Input: part model. Units: mm. Frame: model coordinates. Give positions to 0.01 mm unless a question says otherwise; leave off trailing zeros. Loops run counter-clockwise (first coordinate to the right, second up) from the corner with the lowest first, then second, coordinate; pieces in that order, holes last.
Autodesk Inventor part; units mm, degrees
ref_plane "YZ Plane" through (0, 0, 0) normal (1, 0, 0) x (0, 1, 0)
ref_plane "XZ Plane" through (0, 0, 0) normal (0, 1, 0) x (-1, 0, 0)
ref_plane "XY Plane" through (0, 0, 0) normal (0, 0, 1) x (1, 0, 0)
sketch "main" plane through (0, 0, 0) normal (0, 0, 1) x (1, 0, 0)
  arc A0 (7.9061, 59.9189) -> (2.6576, 57.1432) centre (7.9061, 53.5689) ccw
  line L0 (7.9061, 59.9189) -> (15.7951, 59.9189)
  arc A1 (20.9767, 57.2396) -> (15.7951, 59.9189) centre (15.7951, 53.5689) ccw
  circle A2 centre (15.7951, 53.5689) radius 2.1844
  arc A3 (-27.1814, 13.3264) -> (-31.4423, -3.6797) centre (-6.1872, -0.9705) ccw
  circle A4 centre (15.7951, -9.9311) radius 2.1844
  line L1 (20.9767, 57.2396) -> (20.9767, -12.9584)
  circle A5 centre (-20.2983, -22.6311) radius 2.0955
  line L2 (-2.1836, -39.0438) -> (-15.8326, -52.5455)
  circle A6 centre (-20.2983, -48.0311) radius 2.0955
  line L3 (-31.4423, -3.6797) -> (-26.6121, -48.7084)
  arc A7 (-26.6121, -48.7084) -> (-15.8326, -52.5455) centre (-20.2983, -48.0311) ccw
  line L4 (-27.1814, 13.3264) -> (2.6576, 57.1432)
  line L5 (-1.2414, -14.3873) -> (-1.2414, -36.7866)
  arc A8 (20.637, -14.3873) -> (20.9767, -12.9584) centre (17.8017, -12.9584) ccw
  arc A9 (-2.1836, -39.0438) -> (-1.2414, -36.7866) centre (-4.4164, -36.7866) ccw
  line L6 (20.637, -14.3873) -> (-1.2414, -14.3873)
  point P0 (-2.1335, 12.2772)
  point P1 (20.9767, -16.1334)
  dimension "d0" = 12.7
  dimension "d1" = 6.35
  dimension "d2" = 25.4
  dimension "d3" = 4.191
  dimension "d4" = 4.191
  dimension "d5" = 4.3688
  dimension "d8" = 3.175
sketch "Sketch1" plane through (0, 0, 0) normal (0, 0, 1) x (1, 0, 0)
  arc A0 (-6.35, -7.889) -> (-3.5742, -13.1375) centre (0, -7.889) ccw
  line L0 (-6.35, -7.889) -> (-6.35, 0)
  arc A1 (-3.6706, 5.1816) -> (-6.35, 0) centre (0, 0) ccw
  circle A2 centre (0, 0) radius 2.1844
  arc A3 (40.2425, -42.9766) -> (57.2486, -47.2375) centre (54.5395, -21.9824) ccw
  circle A4 centre (63.5, 0) radius 2.1844
  line L1 (-3.6706, 5.1816) -> (66.5273, 5.1816)
  circle A5 centre (76.2, -36.0934) radius 2.0955
  line L2 (92.6127, -17.9787) -> (106.1144, -31.6277)
  circle A6 centre (101.6, -36.0934) radius 2.0955
  line L3 (57.2486, -47.2375) -> (102.2773, -42.4072)
  arc A7 (102.2773, -42.4072) -> (106.1144, -31.6277) centre (101.6, -36.0934) ccw
  line L4 (40.2425, -42.9766) -> (-3.5742, -13.1375)
  line L5 (67.9562, -17.0366) -> (90.3555, -17.0366)
  arc A8 (67.9562, 4.8419) -> (66.5273, 5.1816) centre (66.5273, 2.0066) ccw
  arc A9 (92.6127, -17.9787) -> (90.3555, -17.0366) centre (90.3555, -20.2116) ccw
  line L6 (67.9562, 4.8419) -> (67.9562, -17.0366)
  point P0 (0, 0)
extrude "Extrusion1" add sketch "Sketch1" along normal blind 1.5875
equation "\"BendRadius\" = Thickness"
equation "\"BendReliefWidth\" = Thickness"
equation "\"BendReliefDepth\" = 0.5 * Thickness"
equation "\"CornerReliefSize\" = 4 * Thickness"
equation "\"MinimumRemnant\" = 2 * Thickness"
equation "\"TransitionRadius\" = BendRadius"
equation "\"JacobiRadiusSize\" = BendRadius"
equation "\"GapSize\" = Thickness"
properties part number "sled" material "Acetal Resin, White"
(1) Cut plane C-C (x = 63.5). Return the cut outline in (y, z).
Values follow:
outline: (-46.57, 0) - (-2.18, 0) - (-2.18, 1.59) - (-46.57, 1.59) - close; (2.18, 0) - (5.18, 0) - (5.18, 1.59) - (2.18, 1.59) - close
(2) Mould query, pull axis X, two halves, no side actions, for faces 1 (the cylindrical face through (65.584, -0.656, 0.783)), 2 (the flat face through (50, -21, 0)), 3 (the cylindrical face through (107.615, -38.129, 0.783)). Classes: +X half, -X half, draft (parallel to the pull), parting line (faces both ways), or undercut.
Values follow:
face 1: undercut
face 2: draft
face 3: +X half
(3) Cut plane B-B (z = 1.3). Return the cut outline in (x, y).
Values follow:
outline: (-6.35, -7.89) arc R6.35 ccw to (-3.57, -13.14) - (40.24, -42.98) arc R25.4 ccw to (57.25, -47.24) - (102.28, -42.41) arc R6.35 ccw to (106.11, -31.63) - (92.61, -17.98) arc R3.17 ccw to (90.36, -17.04) - (67.96, -17.04) - (67.96, 4.84) arc R3.17 ccw to (66.53, 5.18) - (-3.67, 5.18) arc R6.35 ccw to (-6.35, 0) - close; hole circle Ø4.37 at (0, 0); hole circle Ø4.37 at (63.5, 0); hole circle Ø4.19 at (76.2, -36.09); hole circle Ø4.19 at (101.6, -36.09)
(4) Cut plane D-D (y = -20). Return the cut outline in (x, z).
Values follow:
outline: (6.5, 0) - (94.61, 0) - (94.61, 1.59) - (6.5, 1.59) - close
(5) Ray query, probe 1 along X at (y, z) = (-2, 1.15); probe 2 along Y at (x, z) = (75, 0.85); probe 3 along Y at (x, z) = (53.5, 1). Return the intervals inside material, ascending.
Values follow:
probe 1: x = -6.35 to -0.88, 0.88 to 62.62, 64.38 to 67.96
probe 2: y = -45.33 to -37.81, -34.38 to -17.04
probe 3: y = -47.36 to 5.18
(6) Pin query (flat end, axial travel): pin 1 Ø4 at (x, y) = (0, 0) entering from -Z; pin 2 Ø0.8 at (x, z) = (78.5, 0.5) entering from +Y. Return the tip coordinate at first contact, or that it passes through.
Values follow:
pin 1: passes through
pin 2: stops at y = -17.04
(7) Cut plane A-A (x = 76.2). Return the cut outline in (y, z).
Values follow:
outline: (-45.2, 0) - (-38.19, 0) - (-38.19, 1.59) - (-45.2, 1.59) - close; (-34, 0) - (-17.04, 0) - (-17.04, 1.59) - (-34, 1.59) - close
